Check sheet for the modelled part. Datum: model origin and axes. Units: mm. A direction names the side the tool comes from. Give positions to 0.01 mm unless a question says otherwise; leave off trailing zeros. Order: outer loops, then holes, each group sorted by start corner. A loop starts at its lowest first (then second) coordinate and runs counter-clockwise, first axis right, second up.
```python
from build123d import *

# Parameters (mm, degrees)
SKETCH_W        = 80
SKETCH_H        = 60
PAD_DEPTH       = 35
SKETCH001_W     = 72.5
SKETCH001_H     = 52.5
SKETCH001_R     = 3
SKETCH001_R_2   = 1.5
POCKET_DEPTH    = 30
SKETCH002_R     = 1.5
POCKET001_DEPTH = 35.001
SKETCH003_W     = 72.5
SKETCH003_H     = 52.5
POCKET002_DEPTH = 26
FILLET_R        = 3


with BuildPart() as part:
    # Sketch → Pad (new body)
    with BuildSketch(Plane.XY):
        Rectangle(SKETCH_W, SKETCH_H)
    extrude(amount=PAD_DEPTH)

    # Sketch001 (on DatumPlane) → Pocket (cut)
    with BuildSketch(Plane.XY.offset(35)):
        Rectangle(SKETCH001_W, SKETCH001_H)
        with Locations((-32.5, 22.5)):
            Circle(SKETCH001_R, mode=Mode.SUBTRACT)
        with Locations((32.5, 22.5)):
            Circle(SKETCH001_R, mode=Mode.SUBTRACT)
        with Locations((32.5, -22.5)):
            Circle(SKETCH001_R, mode=Mode.SUBTRACT)
        with Locations((-32.5, -22.5)):
            Circle(SKETCH001_R, mode=Mode.SUBTRACT)
        with Locations((-32.5, 22.5)):
            Circle(SKETCH001_R_2)
        with Locations((32.5, 22.5)):
            Circle(SKETCH001_R_2)
        with Locations((32.5, -22.5)):
            Circle(SKETCH001_R_2)
        with Locations((-32.5, -22.5)):
            Circle(SKETCH001_R_2)
    extrude(amount=-POCKET_DEPTH, mode=Mode.SUBTRACT)

    # Sketch002 (on DatumPlane) → Pocket001 (cut, through all)
    with BuildSketch(Plane.XY.offset(35)):
        with Locations((37.5, -27.5)):
            Circle(SKETCH002_R)
        with Locations((37.5, 27.5)):
            Circle(SKETCH002_R)
        with Locations((-37.5, 27.5)):
            Circle(SKETCH002_R)
        with Locations((-37.5, -27.5)):
            Circle(SKETCH002_R)
    extrude(amount=-POCKET001_DEPTH, mode=Mode.SUBTRACT)

    # Sketch003 (on DatumPlane) → Pocket002 (cut)
    with BuildSketch(Plane.XY.offset(35)):
        Rectangle(SKETCH003_W, SKETCH003_H)
    extrude(amount=-POCKET002_DEPTH, mode=Mode.SUBTRACT)

    # Fillet
    fillet_edges = [part.edges().sort_by_distance(p)[0] for p in [
        (-40, -30, 17.5),
        (40, -30, 17.5),
        (40, 30, 17.5),
        (-40, 30, 17.5),
    ]]
    fillet(fillet_edges, radius=FILLET_R)


solid = part.part
```
(1) Release check for a two-part mould opening along X. For faces 1 (the face through (-40, 0, 17)), 2 (the face through (-3, 27, 35)), 3 (the face through (-36.25, 0, 20)) record: released by +X, released by -X, zero draft, split by the parting line, or undercut.
Response values:
face 1: released by -X
face 2: zero draft
face 3: undercut
(2) Material ranges on L1, parallel to X at y = -19.5, z = 10; L2, parallel to Y at x = 25, z = 18.5; L3, parallel to Y at x = -32, z = 7, recorded low to high.
Response values:
L1: x = -40 to -36.25, 36.25 to 40
L2: y = -30 to -26.25, 26.25 to 30
L3: y = -30 to -26.25, -25.46 to -23.91, -21.09 to -19.54, 19.54 to 21.09, 23.91 to 25.46, 26.25 to 30
(3) Cross-section at D-D on x = 32.5. Enter the section's corners in (y, z).
Response values:
outline: (-30, 0) - (30, 0) - (30, 35) - (26.25, 35) - (26.25, 5) - (25.5, 5) - (25.5, 9) - (24, 9) - (24, 5) - (21, 5) - (21, 9) - (19.5, 9) - (19.5, 5) - (-19.5, 5) - (-19.5, 9) - (-21, 9) - (-21, 5) - (-24, 5) - (-24, 9) - (-25.5, 9) - (-25.5, 5) - (-26.25, 5) - (-26.25, 35) - (-30, 35) - close
(4) Cross-section at B-B on x = -24.5. Enter the section's corners in (y, z).
Response values:
outline: (-30, 0) - (30, 0) - (30, 35) - (26.25, 35) - (26.25, 5) - (-26.25, 5) - (-26.25, 35) - (-30, 35) - close
(5) Cross-section at C-C on y = 15.5. Enter the section's corners in (x, z).
Response values:
outline: (-40, 0) - (40, 0) - (40, 35) - (36.25, 35) - (36.25, 5) - (-36.25, 5) - (-36.25, 35) - (-40, 35) - close
(6) Set-up check for faces 4 (the face through (39.14, -29.1, 17.74)), 5 (the face through (-31, -24, 9)): record each of +Z, -Z, +X, -X, +Y, -Y from which the full face is reachable in a straight line by a thin tool's end or side.
Response values:
face 4: +Z, -Z, +X, -Y
face 5: +Z
(7) Gauge pin test, flat ends, axial feed: pin 1 Ø2.5 at (x, y) = (32, -23) entering from +Z; pin 2 Ø1.5 at (x, y) = (-33, -22) entering from +Z. Record the tip position at first contact, or that the pin passes through.
Response values:
pin 1: stops at z = 9
pin 2: stops at z = 5
(8) Cross-section at A-A on z = 19.5. Enter the section's corners in (x, y).
Response values:
outline: (-40, -27) arc R3 ccw to (-37, -30) - (37, -30) arc R3 ccw to (40, -27) - (40, 27) arc R3 ccw to (37, 30) - (-37, 30) arc R3 ccw to (-40, 27) - close; hole circle Ø3 at (-37.5, -27.5); hole circle Ø3 at (-37.5, 27.5); hole (-36.25, -26.25) - (36.25, -26.25) - (36.25, 26.25) - (-36.25, 26.25) - close; hole circle Ø3 at (37.5, -27.5); hole circle Ø3 at (37.5, 27.5)
